Geometry: final body of the model. Coordinates: model frame, mm. Face numbers are marked on the shaded views. Coordinates: 2 decimals unless noted, no trailing zeros. Loops run counter-clockwise (first coordinate to the right, second up) from the corner with the lowest first, then second, coordinate; pieces in that order, holes last. Notation, with made-up numbers: (59, -10.5) - (81, -10.5) arc R25 cw to (81, 20.5) - close; hole circle Ø2 at (67.5, -32). An arc over 180 degrees is marked (long way). Answer in a Markdown table with one row per item.
from build123d import *

# Parameters (mm, degrees)
SKETCH1_W           = 45
SKETCH1_H           = 4
BOSS_EXTRUDE1_DEPTH = 18
SKETCH2_R           = 8.5
CUT_EXTRUDE2_DEPTH  = 0.5
SKETCH3_R           = 3
CUT_EXTRUDE3_DEPTH  = 4.5
SKETCH4_R           = 2.5
CUT_EXTRUDE4_DEPTH  = 5
SKETCH6_R           = 0.8
CUT_EXTRUDE6_DEPTH  = 4.5
FILLET1_R           = 10
SKETCH7_R           = 4
CUT_EXTRUDE7_DEPTH  = 1.555
CUT_EXTRUDE8_DEPTH  = 1.3
SKETCH9_R           = 0.9
CUT_EXTRUDE9_DEPTH  = 5
SKETCH10_R          = 0.9
CUT_EXTRUDE10_DEPTH = 5
CHAMFER1_SIZE       = 0.7


with BuildPart() as part:
    # Sketch1 → Boss-Extrude1 (new body)
    with BuildSketch(Plane(origin=(0, 0, 0), x_dir=(1, 0, 0), z_dir=(0, 1, 0))):
        with Locations((-22.5, 2)):
            Rectangle(SKETCH1_W, SKETCH1_H)
    extrude(amount=BOSS_EXTRUDE1_DEPTH)

    # Sketch2 → Cut-Extrude2 (cut)
    with BuildSketch(Plane.XY):
        with Locations((-22.5, 9)):
            Circle(SKETCH2_R)
    extrude(amount=-CUT_EXTRUDE2_DEPTH, mode=Mode.SUBTRACT)

    # Sketch3 → Cut-Extrude3 (cut, through all)
    with BuildSketch(Plane.XY.offset(-0.5)):
        with Locations((-22.5, 9)):
            Circle(SKETCH3_R)
    extrude(amount=-CUT_EXTRUDE3_DEPTH, mode=Mode.SUBTRACT)

    # Sketch4 → Cut-Extrude4 (cut, through all)
    with BuildSketch(Plane.XY):
        with Locations((-35.5, 9)):
            Circle(SKETCH4_R)
        with Locations((-9.5, 9)):
            Circle(SKETCH4_R)
    extrude(amount=-CUT_EXTRUDE4_DEPTH, mode=Mode.SUBTRACT)

    # Sketch6 → Cut-Extrude6 (cut, through all)
    with BuildSketch(Plane.XY.offset(-0.5)):
        with Locations((-18.169872981, 11.5)):
            Circle(SKETCH6_R)
        with Locations((-18.169872981, 6.5)):
            Circle(SKETCH6_R)
        with Locations((-26.830127019, 6.5)):
            Circle(SKETCH6_R)
        with Locations((-26.830127019, 11.5)):
            Circle(SKETCH6_R)
    extrude(amount=-CUT_EXTRUDE6_DEPTH, mode=Mode.SUBTRACT)

    # Fillet1
    fillet1_edges = [part.edges().sort_by_distance(p)[0] for p in [
        (-45, 18, -2),
        (0, 18, -2),
    ]]
    fillet(fillet1_edges, radius=FILLET1_R)

    # Sketch7 → Cut-Extrude7 (cut)
    with BuildSketch(Plane.XY):
        with Locations((-35.5, 9)):
            Circle(SKETCH7_R)
        with Locations((-9.5, 9)):
            Circle(SKETCH7_R)
    extrude(amount=-CUT_EXTRUDE7_DEPTH, mode=Mode.SUBTRACT)

    # Sketch8 → Cut-Extrude8 (cut)
    with BuildSketch(Plane.XZ):
        Polygon((-5.217293911, -2), (-4.417293911, -0.614359354), (-2.817293911, -0.614359354), (-2.017293911, -2), (-2.817293911, -3.385640646), (-4.417293911, -3.385640646), align=None)
        Polygon((-39.782706089, -2), (-40.582706089, -0.614359354), (-42.182706089, -0.614359354), (-42.982706089, -2), (-42.182706089, -3.385640646), (-40.582706089, -3.385640646), align=None)
    extrude(amount=-CUT_EXTRUDE8_DEPTH, mode=Mode.SUBTRACT)

    # Sketch9 → Cut-Extrude9 (cut)
    with BuildSketch(Plane.XZ.offset(-1.3)):
        with Locations((-41.382706089, -2)):
            Circle(SKETCH9_R)
    extrude(amount=-CUT_EXTRUDE9_DEPTH, mode=Mode.SUBTRACT)

    # Sketch10 → Cut-Extrude10 (cut)
    with BuildSketch(Plane.XZ.offset(-1.3)):
        with Locations((-3.617293911, -2)):
            Circle(SKETCH10_R)
    extrude(amount=-CUT_EXTRUDE10_DEPTH, mode=Mode.SUBTRACT)

    # Chamfer1
    chamfer1_edges = [part.edges().sort_by_distance(p)[0] for p in [
        (-27.630127019, 11.5, -4),
        (-18.969872981, 11.5, -4),
        (-18.969872981, 6.5, -4),
        (-27.630127019, 6.5, -4),
    ]]
    chamfer(chamfer1_edges, length=CHAMFER1_SIZE)


solid = part.part
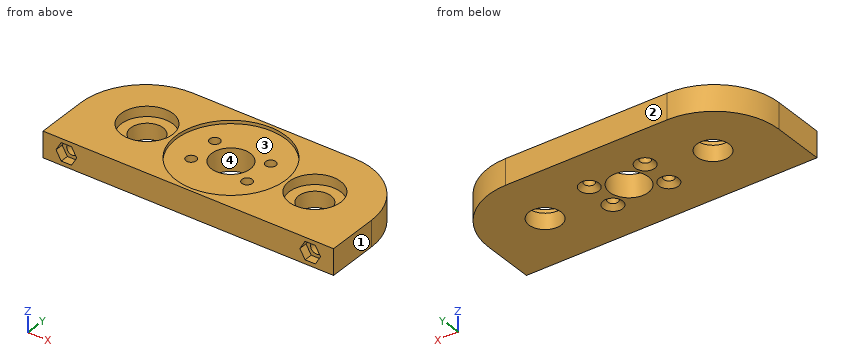
(1) First-contact query: pin 1 Ø2 at (x, z) = (-3.62, -2) entering from +Y; pin 2 Ø2.5 at (x, y) = (-18.17, 11.5) entering from +Z; pin 3 Ø6.5 at (x, y) = (-35.5, 9) entering from -Z; pin 4 Ø1.1 at (x, z) = (-41.38, -2) entering from +Y. Flat tips, straight axial feed; report the tip coordinate or a pass-through.
Verdict:
| item | result |
|---|---|
| pin 1 | stops at y = 16.43 |
| pin 2 | stops at z = -0.5 |
| pin 3 | stops at z = -4 |
| pin 4 | stops at y = 16.12 |
(2) Cut plane B-B on y = 2.25. Output: boundary loops of the cut face in (x, z).
Verdict:
| item | result |
|---|---|
| outline | (-45, -4) - (0, -4) - (0, 0) - (-17.33, 0) - (-17.33, -0.5) - (-27.67, -0.5) - (-27.67, 0) - (-45, 0) - close; hole circle Ø1.8 at (-41.38, -2); hole circle Ø1.8 at (-3.62, -2) |
(3) Ray query, probe 1 along X at (y, z) = (5.5, -0.8); probe 2 along Z at (x, y) = (-11.5, 12) (3 decimals); probe 3 along Z at (x, y) = (-17, 4.5). Return the intervals inside material, ascending.
Verdict:
| item | result |
|---|---|
| probe 1 | x = -45 to -37.44, -33.56 to -11.44, -7.56 to 0 |
| probe 2 | z = -4 to -1.555 |
| probe 3 | z = -4 to -0.5 |
(4) Pull-direction query (X, two-part tool) for the marked faces 1, 2, 3 and 4; classes: pulls with the +X half, pulls with the -X half, needs draft (parallel to the pull), parting line crosses it, or undercut.
Verdict:
| item | result |
|---|---|
| face 1 | pulls with the +X half |
| face 2 | needs draft |
| face 3 | undercut |
| face 4 | undercut |
(5) Cut plane D-D on y = 13.75. Output: boundary loops of the cut face in (x, z), then the cut area to 3 significant figures.
Verdict:
| item | result |
|---|---|
| outline | (-43.18, -4) - (-1.82, -4) - (-1.82, 0) - (-15.45, 0) - (-15.45, -0.5) - (-29.55, -0.5) - (-29.55, 0) - (-43.18, 0) - close |
| area | 158 mm² |
(6) Cut plane A-A on x = -22.5. Output: boundary loops of the cut face in (y, z), then the cut area to 3 significant figures.
Verdict:
| item | result |
|---|---|
| outline | (0, -4) - (6, -4) - (6, -0.5) - (0.5, -0.5) - (0.5, 0) - (0, 0) - close; (12, -4) - (18, -4) - (18, 0) - (17.5, 0) - (17.5, -0.5) - (12, -0.5) - close |
| area | 42.5 mm² |
(7) Cut plane C-C on x = -41.5. Output: boundary loops of the cut face in (y, z).
Verdict:
| item | result |
|---|---|
| outline | (0, -4) - (15.6, -4) - (15.6, 0) - (0, 0) - (0, -0.61) - (1.3, -0.61) - (1.3, -1.11) - (6.3, -1.11) - (6.3, -2.89) - (1.3, -2.89) - (1.3, -3.39) - (0, -3.39) - close |
